Work out the finished part from the listing and answer in its coordinate system (mm). A direction names the side the tool comes from. Round coordinates to 2 decimals unless told otherwise and drop trailing zeros. Order: outer loops, then holes, each group sorted by start corner. A loop starts at its lowest first (then second) coordinate and runs counter-clockwise, first axis right, second up. Notation, with made-up numbers: (-9.5, 2.25) - (8.5, 2.25) arc R29 cw to (8.5, 34.25) - close; hole circle Ø2 at (28.25, 12.5). An arc over 180 degrees is marked (long way). Use CSV: the item, a comma, the result in double quotes.
from build123d import *

# Parameters (mm, degrees)
SKETCH_1_W          = 43
SKETCH_1_H          = 45
SKETCH_1_R          = 1
SKETCH_1_W_2        = 9
SKETCH_1_H_2        = 9
EXTRUDE_1_DEPTH     = 2
SKETCH_3_W          = 17
SKETCH_3_H          = 45
EXTRUDE_3_DEPTH     = 1.5
EXTRUDE_4_DEPTH     = 6
SKETCH_1_3_R        = 1
EXTRUDE_5_DEPTH     = 6
SKETCH_6_R          = 1.4
CUT_EXTRUDE_1_DEPTH = 37.421147703
CHAMFER_1_SIZE      = 2
SKETCH_7_W          = 12
SKETCH_7_H          = 25.2
EXTRUDE_6_DEPTH     = 2
FILLET_1_R          = 5


with BuildPart() as part:
    # Sketch 1 → Extrude 1 (new body)
    with BuildSketch(Plane.XY):
        with Locations((-6, 0)):
            Rectangle(SKETCH_1_W, SKETCH_1_H)
        with Locations((-6, -10.5)):
            Circle(SKETCH_1_R, mode=Mode.SUBTRACT)
        with Locations((-6, 0)):
            Rectangle(SKETCH_1_W_2, SKETCH_1_H_2, mode=Mode.SUBTRACT)
        with Locations((6, -10.5)):
            Circle(SKETCH_1_R, mode=Mode.SUBTRACT)
        with Locations((-6, 10.5)):
            Circle(SKETCH_1_R, mode=Mode.SUBTRACT)
        with Locations((6, 10.5)):
            Circle(SKETCH_1_R, mode=Mode.SUBTRACT)
    extrude(amount=EXTRUDE_1_DEPTH)

    # Sketch 3 → Extrude 3 (add)
    with BuildSketch(Plane.XY.offset(2)):
        with Locations((-19, 0)):
            Rectangle(SKETCH_3_W, SKETCH_3_H)
    extrude(amount=EXTRUDE_3_DEPTH)

    # Sketch 4 → Extrude 4 (add)
    with BuildSketch(Plane.XY.offset(2)):
        Polygon((-15.5, -22.5), (15.5, -22.5), (15.5, 22.5), (-15.5, 22.5), (-27.5, 22.5), (-27.5, 12.6), (-15.5, 12.6), (8.9, 12.6), (8.9, -12.6), (-15.5, -12.6), (-27.5, -12.6), (-27.5, -22.5), align=None)
    extrude(amount=EXTRUDE_4_DEPTH)

    # Sketch 1_3 → Extrude 5 (add)
    with BuildSketch(Plane.XY):
        with Locations((-6, 10.5)):
            Circle(SKETCH_1_3_R)
        with Locations((6, 10.5)):
            Circle(SKETCH_1_3_R)
        with Locations((-6, -10.5)):
            Circle(SKETCH_1_3_R)
        with Locations((6, -10.5)):
            Circle(SKETCH_1_3_R)
    extrude(amount=EXTRUDE_5_DEPTH)

    # Sketch 6 → Cut-Extrude 1 (cut, through all)
    with BuildSketch(Plane.XY):
        with Locations((-10, 17.5)):
            Circle(SKETCH_6_R)
        with Locations(Location((10, 17.5, 0), (0, 0, 180))):
            Circle(SKETCH_6_R)
        with Locations((10, -17.5)):
            Circle(SKETCH_6_R)
        with Locations(Location((-10, -17.5, 0), (0, 0, 180))):
            Circle(SKETCH_6_R)
    extrude(amount=CUT_EXTRUDE_1_DEPTH, mode=Mode.SUBTRACT)

    # Chamfer 1
    chamfer_1_edges = [part.edges().sort_by_distance(p)[0] for p in [
        (-8.6, -17.5, 0),
        (8.6, -17.5, 0),
        (11.4, 17.5, 0),
        (-11.4, 17.5, 0),
    ]]
    chamfer(chamfer_1_edges, length=CHAMFER_1_SIZE)

    # Sketch 7 → Extrude 6 (add)
    with BuildSketch(Plane.XY.offset(3.5)):
        with Locations((-21.5, 0)):
            Rectangle(SKETCH_7_W, SKETCH_7_H)
    extrude(amount=EXTRUDE_6_DEPTH)

    # Fillet 1
    fillet_1_edges = [part.edges().sort_by_distance(p)[0] for p in [
        (-27.5, 22.5, 4),
        (15.5, 22.5, 4),
        (15.5, -22.5, 4),
        (-27.5, -22.5, 4),
    ]]
    fillet(fillet_1_edges, radius=FILLET_1_R)


solid = part.part
(1) Find section C-C (z = 7). Determine the outline of the cut face in (x, y), and give its area (3 significant figures).
Findings below:
outline,"(-27.5, -17.5) arc R5 ccw to (-22.5, -22.5) - (10.5, -22.5) arc R5 ccw to (15.5, -17.5) - (15.5, 17.5) arc R5 ccw to (10.5, 22.5) - (-22.5, 22.5) arc R5 ccw to (-27.5, 17.5) - (-27.5, 12.6) - (8.9, 12.6) - (8.9, -12.6) - (-27.5, -12.6) - close; hole circle Ø2.8 at (-10, -17.5); hole circle Ø2.8 at (-10, 17.5); hole circle Ø2.8 at (10, -17.5); hole circle Ø2.8 at (10, 17.5)"
area,"972 mm²"
(2) For faces 1 (the flat face through (-6, 4.5, 1)), 2 (the flat face through (-22, 0, 5.5)), 3 (the cylindrical face through (-6.737, 11.176, 3.972)), determine the directions among +Z, -Z, +X, -X, +Y, -Y from which every point of the face is accessible in a straight line to the end or side of a thin tool.
Findings below:
face 1,"+Z, -Z"
face 2,"+Z, -X"
face 3,"+Z"
(3) The mould has two halves that part along Y. Classify faces 4 (the flat face through (-6, -22.5, 4)), 5 (the flat face through (-1, 0, 2)), 6 (the flat face through (6, -10, 6)), 7 (the flat face through (15.5, 0, 4)): released by +Y, released by -Y, zero draft, split by the parting line, or undercut.
Findings below:
face 4,"released by -Y"
face 5,"undercut"
face 6,"undercut"
face 7,"zero draft"
(4) Each of these flat-tipped pins is pushed along its axis until it touches: pin 1 (1.7 mm diameter, centred on x = 10, y = -17.5, fed in from -Z); pin 2 (3.5 mm diameter, centred on x = -10, y = 17.5, fed in from -Z); pin 3 (2.5 mm diameter, centred on x = -14, y = -1, fed in from +Z); pin 4 (1.6 mm diameter, centred on x = -6, y = -10, fed in from +Z). Where does it stop, or does it pass through?
Findings below:
pin 1,"passes through"
pin 2,"stops at z = 1.65"
pin 3,"stops at z = 3.5"
pin 4,"stops at z = 6"
(5) Find the intervals of material crossed by L1, parallel to X at y = -17.5, z = 5.85; L2, parallel to Y at x = -10, z = 4.4; L3, parallel to Y at x = 10, z = 5.65, in increasing order. Write a range as from..to.
Findings below:
L1,"x = -27.5..-11.4, -8.6..8.6, 11.4..15.5"
L2,"y = -22.5..-18.9, -16.1..-12.6, 12.6..16.1, 18.9..22.5"
L3,"y = -22.5..-18.9, -16.1..16.1, 18.9..22.5"
(6) Find section A-A (z = 2.75). State how many separate pieces and enclosed holes the cut face has, and give its area (3 significant figures).
Findings below:
separate pieces,"5"
enclosed holes,"5"
area,"1,410 mm²"
(7) Find section B-B (x = -6). Determine the outline of the cut face in (y, z), and give its area (3 significant figures).
Findings below:
outline,"(-22.5, 0) - (-4.5, 0) - (-4.5, 2) - (-9.5, 2) - (-9.5, 6) - (-11.5, 6) - (-11.5, 2) - (-12.6, 2) - (-12.6, 8) - (-22.5, 8) - close; (4.5, 0) - (22.5, 0) - (22.5, 8) - (12.6, 8) - (12.6, 2) - (11.5, 2) - (11.5, 6) - (9.5, 6) - (9.5, 2) - (4.5, 2) - close"
area,"207 mm²"
(8) Find section D-D (y = -10.5). Determine the outline of the cut face in (x, z).
Findings below:
outline,"(-27.5, 0) - (15.5, 0) - (15.5, 8) - (8.9, 8) - (8.9, 2) - (7, 2) - (7, 6) - (5, 6) - (5, 2) - (-5, 2) - (-5, 6) - (-7, 6) - (-7, 2) - (-10.5, 2) - (-10.5, 3.5) - (-15.5, 3.5) - (-15.5, 5.5) - (-27.5, 5.5) - close"
